Part model, mm, in its own coordinate system. Coordinates: 2 decimals unless noted, no trailing zeros. Order: outer loops, then holes, each group sorted by start corner. A loop starts at its lowest first (then second) coordinate and runs counter-clockwise, first axis right, second up.
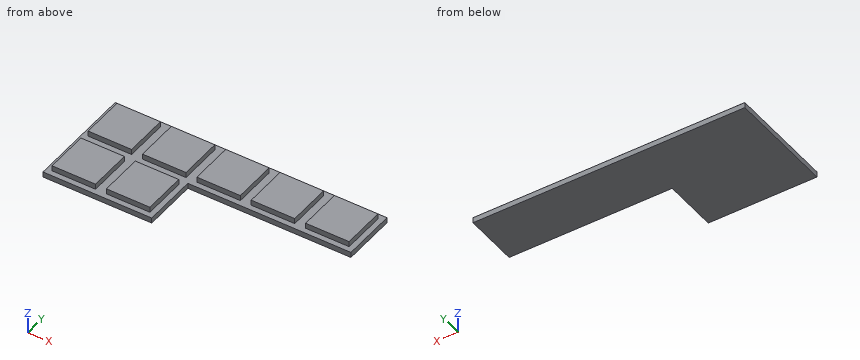
from build123d import *

# Parameters (mm, degrees)
F1_DEPTH = 1
F2_W     = 8
F2_H     = 8
F3_DEPTH = 1


# Not quite as in the source:
# - a feature names something its author has since deleted; it is built from what else it names


with BuildPart() as f1:
    # F0 (on Top) → F1 (new body)
    with BuildSketch(Plane.XY):
        Polygon((30, 10), (-20, 10), (-20, -10), (0, -10), (0, 0), (30, 0), align=None)
    extrude(amount=F1_DEPTH)

    # F2 (on face) → F3 (join)
    with BuildSketch(Plane.XY.offset(1)):
        with Locations((-15, 5)):
            Rectangle(F2_W, F2_H)
        with Locations((-15, -5)):
            Rectangle(F2_W, F2_H)
        with Locations((-5, -5)):
            Rectangle(F2_W, F2_H)
        with Locations((-5, 5)):
            Rectangle(F2_W, F2_H)
        with Locations((5, 5)):
            Rectangle(F2_W, F2_H)
        with Locations((15, 5)):
            Rectangle(F2_W, F2_H)
        with Locations((25, 5)):
            Rectangle(F2_W, F2_H)
    extrude(amount=F3_DEPTH)


solid = f1.part
Q1. Pin check, flat tips, straight feed: pin 1 Ø1.1 at (y, z) = (-3.5, 1.5) entering from -X; pin 2 Ø0.8 at (x, z) = (27, 1.5) entering from -Y; pin 3 Ø0.8 at (x, z) = (27, 1.5) entering from +Y; pin 4 Ø0.8 at (y, z) = (5.5, 1.5) entering from -X. Stop position of each tip, or through.
Results list:
pin 1: stops at x = -20
pin 2: stops at y = 1
pin 3: stops at y = 9
pin 4: stops at x = -19
Q2. Wall check: line 1 along X through (y, z) = (4, 1.45); line 2 along Y through (x, z) = (-16.5, 1.7); line 3 along X through (y, z) = (-5, 1.4). Give the ranges that are in metal, low to high.
Results list:
line 1: x = -19 to -11, -9 to -1, 1 to 9, 11 to 19, 21 to 29
line 2: y = -9 to -1, 1 to 9
line 3: x = -19 to -11, -9 to -1
Q3. Cut at B-B on y = -7. Write the cut outline in (x, z).
Results list:
outline: (-20, 0) - (0, 0) - (0, 1) - (-1, 1) - (-1, 2) - (-9, 2) - (-9, 1) - (-11, 1) - (-11, 2) - (-19, 2) - (-19, 1) - (-20, 1) - close
Q4. Cut at C-C on x = 16. Write the cut outline in (y, z).
Results list:
outline: (0, 0) - (10, 0) - (10, 1) - (9, 1) - (9, 2) - (1, 2) - (1, 1) - (0, 1) - close
Q5. Cut at A-A on z = 1.5. Write the cut outline in (x, y).
Results list:
outline: (-19, -9) - (-11, -9) - (-11, -1) - (-19, -1) - close; (-19, 1) - (-11, 1) - (-11, 9) - (-19, 9) - close; (-9, -9) - (-1, -9) - (-1, -1) - (-9, -1) - close; (-9, 1) - (-1, 1) - (-1, 9) - (-9, 9) - close; (1, 1) - (9, 1) - (9, 9) - (1, 9) - close; (11, 1) - (19, 1) - (19, 9) - (11, 9) - close; (21, 1) - (29, 1) - (29, 9) - (21, 9) - close
Q6. Cut at D-D on y = 8. Write the cut outline in (x, z), and give its area (3 significant figures).
Results list:
outline: (-20, 0) - (30, 0) - (30, 1) - (29, 1) - (29, 2) - (21, 2) - (21, 1) - (19, 1) - (19, 2) - (11, 2) - (11, 1) - (9, 1) - (9, 2) - (1, 2) - (1, 1) - (-1, 1) - (-1, 2) - (-9, 2) - (-9, 1) - (-11, 1) - (-11, 2) - (-19, 2) - (-19, 1) - (-20, 1) - close
area: 90.0 mm2
